Read the model definition and answer for the solid it produces. Units are mm, in the model's axes. A direction names the side the tool comes from. Coordinates: 2 decimals unless noted, no trailing zeros. Write each loop counter-clockwise with the first axis right and the second up, starting at its lowest first coordinate (ties: lowest second). Pieces come first, ordered by that corner, then holes.
1) Each of these flat-tipped pins is pushed along its axis until it touches: pin 1 Ø23 at (x, y) = (-238.125, 304.8) entering from -Z; pin 2 Ø8 at (x, z) = (135, 16.5) entering from -Y. Where does it stop, or does it pass through?
2) The part is cut by section B-B (z = 7). Give the number of separate pieces and of enclosed holes in the cut face, then the cut area to 3 significant figures.
3) The part is cut by section C-C (x = 73.5). Determine the outline of the cut face in (y, z).
4) Determine the mould class of faces 1 (the face through (-272.406, 339.278, 9.392)), 2 (the face through (-197.347, 319.437, 9.392)), 3 (the face through (-1, 325, 0)), 4 (the face through (210.843, 278.205, 9.392)) for opening direction X: +X half, -X half, draft (parallel to the pull), parting line (faces both ways), or undercut.
5) The part is cut by section A-A (y = 218). Determine the outline of the cut face in (x, z) (3 decimals), then the cut area to 3 significant figures.
6) Which of the six approach directions +Z, -Z, +X, -X, +Y, -Y give full straight-line access (tool end or side, diameter ignored) to faces 5 (the face through (276.225, 163, 9)), 6 (the face through (-3, 323.85, 9)), 7 (the face through (197.15, 319.66, 9.39))?
7) Find the intervals of material crossed by line 1 (X direction, y = 304.8, z = 4) (3 decimals); line 2 (X direction, y = 306.5, z = 8.75) (3 decimals); line 3 (X direction, y = 79, z = 12) (3 decimals), in increasing order.
from build123d import *

# Parameters (mm, degrees)
SKETCH1_R           = 19.05
BOSS_EXTRUDE1_DEPTH = 19.05


with BuildPart() as part:
    # Sketch1 → Boss-Extrude1 (new body)
    with BuildSketch(Plane.XY):
        with BuildLine():
            Line((276.225, 0), (276.225, 330.2))
            ThreePointArc((276.225, 330.2), (272.505256121, 339.180256121), (263.525, 342.9))
            Line((263.525, 342.9), (-263.525, 342.9))
            ThreePointArc((-263.525, 342.9), (-272.505256121, 339.180256121), (-276.225, 330.2))
            Line((-276.225, 330.2), (-276.225, 0))
            Line((-276.225, 0), (-257.175, 0))
            Line((-257.175, 0), (-257.175, 76.2))
            Line((-257.175, 76.2), (-257.175, 165.1))
            Line((-257.175, 165.1), (-257.175, 254.398437524))
            ThreePointArc((-257.175, 254.398437524), (-252.875260413, 263.923437524), (-242.8875, 266.998828143))
            ThreePointArc((-242.8875, 266.998828143), (-211.184231637, 277.859231637), (-200.323828143, 309.5625))
            ThreePointArc((-200.323828143, 309.5625), (-197.248437524, 319.550260413), (-187.723437524, 323.85))
            Line((-187.723437524, 323.85), (187.723437524, 323.85))
            ThreePointArc((187.723437524, 323.85), (197.248437524, 319.550260413), (200.323828143, 309.5625))
            ThreePointArc((200.323828143, 309.5625), (211.184231637, 277.859231637), (242.8875, 266.998828143))
            ThreePointArc((242.8875, 266.998828143), (252.875260413, 263.923437524), (257.175, 254.398437524))
            Line((257.175, 254.398437524), (257.175, 165.1))
            Line((257.175, 165.1), (257.175, 76.2))
            Line((257.175, 76.2), (257.175, 0))
            Line((257.175, 0), (276.225, 0))
        make_face()
        with Locations(Location((238.125, 304.8, 0), (0, 0, 180))):
            Circle(SKETCH1_R, mode=Mode.SUBTRACT)
        with Locations(Location((-238.125, 304.8, 0), (0, 0, 180))):
            Circle(SKETCH1_R, mode=Mode.SUBTRACT)
    extrude(amount=BOSS_EXTRUDE1_DEPTH)


solid = part.part
Reported:
1. pin 1: passes through
1. pin 2: stops at y = 323.85
2. separate pieces: 1
2. enclosed holes: 2
2. area: 26,500 mm2
3. outline: (323.85, 0) - (342.9, 0) - (342.9, 19.05) - (323.85, 19.05) - close
4. face 1: -X half
4. face 2: undercut
4. face 3: draft
4. face 4: undercut
5. outline: (-276.225, 0) - (-257.175, 0) - (-257.175, 19.05) - (-276.225, 19.05) - close; (257.175, 0) - (276.225, 0) - (276.225, 19.05) - (257.175, 19.05) - close
5. area: 726 mm2
6. face 5: +Z, -Z, +X, +Y, -Y
6. face 6: +Z, -Z, -Y
6. face 7: +Z, -Z
7. line 1: x = -276.225 to -257.175, -219.075 to -200.025, 200.025 to 219.075, 257.175 to 276.225
7. line 2: x = -276.225 to -257.099, -219.151 to -200.063, 200.063 to 219.151, 257.099 to 276.225
7. line 3: x = -276.225 to -257.175, 257.175 to 276.225
